Build history of the part. All positions in model axes, mm. Face numbers are marked on the shaded views. A direction names the side the tool comes from. Give positions to 0.01 mm unless a question says otherwise; leave off trailing zeros. Loops run counter-clockwise (first coordinate to the right, second up) from the corner with the lowest first, then second, coordinate; pieces in that order, holes last. Notation, with made-up numbers: M 76,0.25 L 95,0.25 A18 ccw 95,32.25 Z; hole C -12,-18 d11. An arc over 180 degrees is marked long. Answer as a JSON object with one key per item and string values. Group by question number.
1. Slice it at D-D (y = 1.8). Give the number of separate pieces and of enclosed holes in the cut face, then the cut area to 3 significant figures.
2. Drill centre lines: line 1 along X through (y, z) = (1.05, 11); line 2 along X through (y, z) = (2.75, 8.25); line 3 along Z through (x, y) = (-0.25, 2.3). Where is each one in solid material? Low to high. Write a range as [from, to].
3. Drop flat-ended pins along their axis: pin 1 Ø8 at (x, z) = (-3.5, -11.5) entering from -Y; pin 2 Ø1.5 at (x, y) = (-6, 0.5) entering from -Z; pin 3 Ø1.5 at (y, z) = (1.5, -7.5) entering from -X; pin 4 Ø1.5 at (x, y) = (-8.5, 1) entering from +Z. Give the stop position or say it passes through.
4. 3-axis set-ups, long thin cutter, end or side, ignore diameter. For the marked faces 4 and 5: which of +Z, -Z, +X, -X, +Y, -Y reach the whole face in a straight line?
5. Slice it at A-A (z = 10.25). List the corners of the cut face in (x, y).
6. Slice it at C-C (x = -11.5). List the corners of the cut face in (y, z), then the cut area to 3 significant figures.
7. Mould opens along X. For the marked faces 1, 2 and 3 say: released by +X, released by -X, zero draft, split by the parting line, or undercut.
8. Slice it at B-B (x = 7.25). List the corners of the cut face in (y, z).
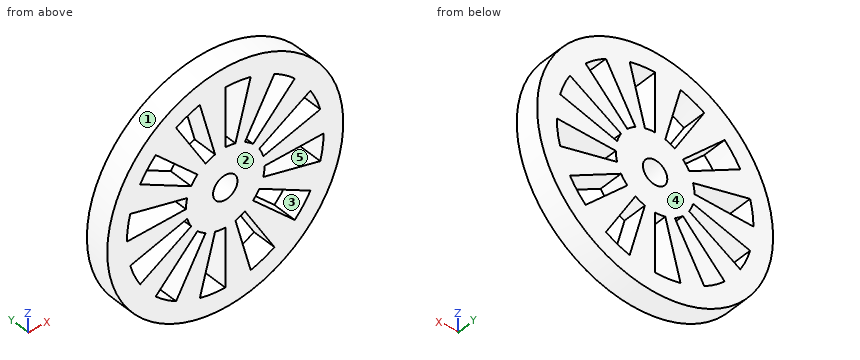
Autodesk Inventor part; units mm, degrees
ref_plane "YZ Plane" through (0, 0, 0) normal (1, 0, 0) x (0, 1, 0)
ref_plane "XZ Plane" through (0, 0, 0) normal (0, 1, 0) x (-1, 0, 0)
ref_plane "XY Plane" through (0, 0, 0) normal (0, 0, 1) x (1, 0, 0)
sketch "草圖1" plane through (0, 0, 0) normal (0, 1, 0) x (-1, 0, 0)
  circle A0 centre (0, 0) radius 15
  line L0 (0, 0) -> (15, 0)
  line L1 (0, 0) -> (7.5, -12.9904)
  line L2 (0, 0) -> (12.9904, -7.5)
  circle A1 centre (0, 0) radius 12.5
  circle A2 centre (0, 0) radius 5
  circle A3 centre (0, 0) radius 1.55
  line L3 (0, 0) -> (10.6066, -10.6066)
  line L4 (0, 0) -> (14.4889, -3.8823)
  point P0 (6.25, -10.8253)
  point P1 (2.5, -4.3301)
  point P2 (4.3301, -2.5)
  point P3 (10.8253, -6.25)
  point P4 (12.0741, -3.2352)
  point P5 (4.8296, -1.2941)
  point P6 (8.8388, -8.8388)
  point P7 (3.5355, -3.5355)
  dimension "d0" = 30
  dimension "d1" = 60
  dimension "d2" = 30
  dimension "d3" = 25
  dimension "d4" = 10
  dimension "d12" = 3.1
  dimension "d15" = 15
  dimension "d16" = 15
extrude "擠出1" add sketch "草圖1" along normal blind 3
extrude "擠出2" cut sketch "草圖1" along normal blind 3 contours L1 A2 L3 A1 | A1 L2 A2 L4
pattern_circular "環形陣列1" count 6 over 360 about axis through (0, -10, 0) along (0, 1, 0) of "擠出2"
extrude "擠出3" cut sketch "草圖1" along normal blind 3 contours A3 L4 L0 | L0 L1 A3 | L1 L3 A3 | A3 L2 L4 | L2 A3 L3
properties part number "wheel_12_hollow"
Established:
{
 "1": {"separate pieces": "1", "enclosed holes": "13", "area": "493 mm^2"},
 "2": {"line 1": "x = [-10.2, -5.94], [-2.95, 0], [2.95, 10.2]", "line 2": "x = [-12.53, -9.39], [-8.25, -4.76], [-2.21, 0], [2.21, 4.76], [8.25, 12.53]", "line 3": "z = [-15, -12.5], [-4.99, -1.53], [1.53, 15]"},
 "3": {"pin 1": "stops at y = 0", "pin 2": "stops at z = -14.05", "pin 3": "stops at x = -13.4", "pin 4": "stops at z = 12.84"},
 "4": {"face 4": "+Z, -Z, +X, -X, +Y", "face 5": "+Y, -Y"},
 "5": {"outline": "M -10.95,0 L -5.92,0 L -5.92,3 L -10.95,3 Z; M -2.75,0 L 0,0 L 0,3 L -2.75,3 Z; M 2.75,0 L 5.92,0 L 5.92,3 L 2.75,3 Z; M 7.15,0 L 10.95,0 L 10.95,3 L 7.15,3 Z"},
 "6": {"outline": "M 0,-9.63 L 3,-9.63 L 3,-4.9 L 0,-4.9 Z; M 0,-3.08 L 3,-3.08 L 3,0 L 0,0 Z; M 0,3.08 L 3,3.08 L 3,9.63 L 0,9.63 Z", "area": "43.1 mm^2"},
 "7": {"face 1": "split by the parting line", "face 2": "zero draft", "face 3": "undercut"},
 "8": {"outline": "M 0,-13.13 L 3,-13.13 L 3,-7.25 L 0,-7.25 Z; M 0,-4.19 L 3,-4.19 L 3,-1.94 L 0,-1.94 Z; M 0,0 L 3,0 L 3,1.94 L 0,1.94 Z; M 0,4.19 L 3,4.19 L 3,7.25 L 0,7.25 Z; M 0,10.18 L 3,10.18 L 3,13.13 L 0,13.13 Z"}
}
